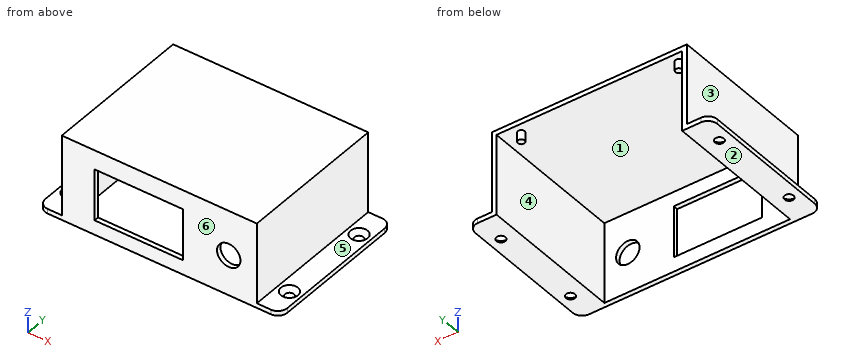
```python
from build123d import *

# Parameters (mm, degrees)
F1_DEPTH       = 80
F0_W           = 99
F0_H           = 43
F0_W_2         = 47
F0_H_2         = 27.5
F0_R           = 6.25
F2_DEPTH       = 2.5
F4_D           = 4.4958
F4_CSINK_D     = 9.1186
F4_CSINK_ANGLE = 82
F5_R           = 5
F6_R           = 1.75
F7_DEPTH       = 5


with BuildPart() as f1:
    # F0 (on Front) → F1 (new body)
    with BuildSketch(Plane.XZ):
        Polygon((-15, -7.75), (-15, 35.25), (84, 35.25), (84, -7.75), (99, -7.75), (99, -5.25), (86.5, -5.25), (86.5, 37.75), (-17.5, 37.75), (-17.5, -5.25), (-30, -5.25), (-30, -7.75), align=None)
    extrude(amount=-F1_DEPTH)

    # F0 (on Front) → F2 (join)
    with BuildSketch(Plane.XZ):
        with Locations((34.5, 13.75)):
            Rectangle(F0_W, F0_H)
        with Locations((23.5, 13.75)):
            Rectangle(F0_W_2, F0_H_2, mode=Mode.SUBTRACT)
        with Locations((71.5, 13.75)):
            Circle(F0_R, mode=Mode.SUBTRACT)
    extrude(amount=-F2_DEPTH)

    # F4 (through all)
    with Locations(Plane.XY.offset(-5.25)):
        with Locations((-23.75, 65), (-23.75, 15), (92.75, 15), (92.75, 65)):
            CounterSinkHole(F4_D / 2, F4_CSINK_D / 2, counter_sink_angle=F4_CSINK_ANGLE)

    # F5
    f5_edges = [f1.edges().sort_by_distance(p)[0] for p in [
        (99, 0, -6.5),
        (-30, 0, -6.5),
        (99, 80, -6.5),
        (-30, 80, -6.5),
    ]]
    fillet(f5_edges, radius=F5_R)

    # F6 (on face) → F7 (join)
    with BuildSketch(Plane(origin=(0, 0, 35.25), x_dir=(1, 0, 0), z_dir=(0, 0, -1))):
        with Locations((-9.5, -75)):
            Circle(F6_R)
        with Locations((74.5, -75)):
            Circle(F6_R)
    extrude(amount=F7_DEPTH)


solid = f1.part
```
Could you check a few things on this model? Use its own coordinates, in mm. Face numbers are marked on the shaded views. A direction names the side the tool comes from. Coordinates: 2 decimals unless noted, no trailing zeros. Loops run counter-clockwise (first coordinate to the right, second up) from the corner with the lowest first, then second, coordinate; pieces in that order, holes last. Notation, with made-up numbers: M 62,-40 L 108,-40 A21 cw 108,-30 Z; hole C -13,2 d1. An arc over 180 degrees is marked long. Put each result on its own line as item: value. Start each with the question number.
(1) Suppose I cut it at C-C on y = 65. Please give me the cut outline in (x, z), then the cut area to 3 significant figures.
(2) Suppose I cut it at D-D on y = 24.5. Please give me the cut outline in (x, z), then the cut area to 4 significant figures.
(3) For the marked faces 4, 5 and 6, which set-ups out of +Z, -Z, +X, -X, +Y, -Y let a thin tool reach every point of the face, with its end or its side?
(4) I need wall thicknesses on line 1 (X direction, y = 6, z = 4); line 2 (Z direction, x = 71.5, y = 1.4); line 3 (X direction, y = 1, z = 13). Which ranges of each line are inside material? Lowest first, please. Write a range as from..to.
(5) Will these pins go through, and if not, where does the flat tip stop? P1, Ø2, axis at x = 75, y = 46, coming from the -Z side; P2, Ø3, axis at x = -9.5, y = 74.5, coming from the -Z side; P3, Ø3, axis at y = 1.5, z = 7.5, coming from the -X side.
(6) Suppose I cut it at B-B on x = -9.5. Please give me the cut outline in (y, z).
(7) Thinking about a two-plate mould opening in X: for the marked faces 1, 2 and 3, which applies, pulls with the +X half, pulls with the -X half, needs draft (parallel to the pull), parting line crosses it, or undercut?
(8) Suppose I cut it at A-A on z = 10. Please give me the cut outline in (x, y).
Solutions:
1. outline: M -30,-7.75 L -26.14,-7.75 L -28.31,-5.25 L -30,-5.25 Z; M -21.36,-7.75 L -15,-7.75 L -15,35.25 L 84,35.25 L 84,-7.75 L 90.36,-7.75 L 88.19,-5.25 L 86.5,-5.25 L 86.5,37.75 L -17.5,37.75 L -17.5,-5.25 L -19.19,-5.25 Z; M 95.14,-7.75 L 99,-7.75 L 99,-5.25 L 97.31,-5.25 Z
1. area: 503 mm2
2. outline: M -30,-7.75 L -15,-7.75 L -15,35.25 L 84,35.25 L 84,-7.75 L 99,-7.75 L 99,-5.25 L 86.5,-5.25 L 86.5,37.75 L -17.5,37.75 L -17.5,-5.25 L -30,-5.25 Z
2. area: 537.5 mm2
3. face 4: -Z, +Y
3. face 5: +Z, +X, +Y, -Y
3. face 6: +Z, -Z, +X, -X, -Y
4. line 1: x = -17.5..-15, 84..86.5
4. line 2: z = -7.75..7.5, 20..37.75
4. line 3: x = -17.5..0, 47..65.3, 77.7..86.5
5. P1: stops at z = 35.25
5. P2: stops at z = 30.25
5. P3: stops at x = -17.5
6. outline: M 0,-7.75 L 2.5,-7.75 L 2.5,35.25 L 73.25,35.25 L 73.25,30.25 L 76.75,30.25 L 76.75,35.25 L 80,35.25 L 80,37.75 L 0,37.75 Z
7. face 1: undercut
7. face 2: needs draft
7. face 3: pulls with the -X half
8. outline: M -17.5,0 L 0,0 L 0,2.5 L -15,2.5 L -15,80 L -17.5,80 Z; M 47,0 L 66.5,0 L 66.5,2.5 L 47,2.5 Z; M 76.5,0 L 86.5,0 L 86.5,80 L 84,80 L 84,2.5 L 76.5,2.5 Z
